from build123d import *

# Parameters (mm, degrees)
ESQUISSE1_W             = 23
ESQUISSE1_H             = 12
BOSS_EXTRU_1_DEPTH      = 21
ESQUISSE2_W             = 4
ESQUISSE2_H             = 11.992585314
BOSS_EXTRU_2_DEPTH      = 1
ESQUISSE3_R             = 0.5
ENL_V_MAT_EXTRU_1_DEPTH = 1
ESQUISSE4_R             = 5.976429807
BOSS_EXTRU_3_DEPTH      = 4
ESQUISSE5_W             = 4.5
ESQUISSE5_H             = 5
BOSS_EXTRU_4_DEPTH      = 3
ENL_V_MAT_EXTRU_3_DEPTH = 32.768695283
ESQUISSE7_R             = 1.5
ENL_V_MAT_EXTRU_4_DEPTH = 3


with BuildPart() as part:
    # Esquisse1 → Boss.-Extru.1 (new body)
    with BuildSketch(Plane(origin=(0, 0, 0), x_dir=(1, 0, 0), z_dir=(0, 1, 0))):
        Rectangle(ESQUISSE1_W, ESQUISSE1_H)
    extrude(amount=BOSS_EXTRU_1_DEPTH)

    # Esquisse2 → Boss.-Extru.2 (add)
    with BuildSketch(Plane(origin=(0, 16, 0), x_dir=(1, 0, 0), z_dir=(0, 1, 0))):
        with Locations((13.5, 0.003707343)):
            Rectangle(ESQUISSE2_W, ESQUISSE2_H)
    boss_extru_2 = extrude(amount=BOSS_EXTRU_2_DEPTH)

    # Esquisse3 → Enlèv. mat.-Extru.1 (cut)
    with BuildSketch(Plane(origin=(0, 17, 0), x_dir=(1, 0, 0), z_dir=(0, 1, 0))):
        with Locations(Location((13.5, 0.003707343, 0), (0, 0, 270))):
            Circle(ESQUISSE3_R)
    enl_v_mat_extru_1 = extrude(amount=-ENL_V_MAT_EXTRU_1_DEPTH, mode=Mode.SUBTRACT)

    # Symétrie1: Boss.-Extru.2 across plane
    add(boss_extru_2.mirror(Plane(origin=(0, 0, 0), x_dir=(0, 0, 1), z_dir=(1, 0, 0))))

    # Symétrie2: Enlèv. mat.-Extru.1 across plane
    add(enl_v_mat_extru_1.mirror(Plane(origin=(0, 0, 0), x_dir=(0, 0, 1), z_dir=(1, 0, 0))), mode=Mode.SUBTRACT)

    # Esquisse4 → Boss.-Extru.3 (add)
    with BuildSketch(Plane(origin=(0, 21, 0), x_dir=(1, 0, 0), z_dir=(0, 1, 0))):
        with Locations(Location((5.523570193, -0.023570193, 0), (0, 0, 270))):
            Circle(ESQUISSE4_R)
    extrude(amount=BOSS_EXTRU_3_DEPTH)

    # Esquisse5 → Boss.-Extru.4 (add)
    with BuildSketch(Plane(origin=(0, 21, 0), x_dir=(1, 0, 0), z_dir=(0, 1, 0))):
        with Locations((-0.452859613, -0.023570193)):
            Rectangle(ESQUISSE5_W, ESQUISSE5_H)
    extrude(amount=BOSS_EXTRU_4_DEPTH)

    # Esquisse6 → Enlèv. mat.-Extru.3 (cut, through all)
    with BuildSketch(Plane.XY.offset(6)):
        Polygon((9.55941942, 0), (11.5, 1.94058058), (11.5, 0), align=None)
    extrude(amount=-ENL_V_MAT_EXTRU_3_DEPTH, mode=Mode.SUBTRACT)

    # Esquisse7 → Enlèv. mat.-Extru.4 (cut)
    with BuildSketch(Plane(origin=(0, 25, 0), x_dir=(1, 0, 0), z_dir=(0, 1, 0))):
        with Locations(Location((5.523570193, -0.023570193, 0), (0, 0, 270))):
            Circle(ESQUISSE7_R)
    extrude(amount=-ENL_V_MAT_EXTRU_4_DEPTH, mode=Mode.SUBTRACT)


solid = part.part
Source: CAD feature listing. Evaluate the final solid. Frame: model axes, mm. A direction names the side the tool comes from. Give positions to 0.01 mm unless a question says otherwise; leave off trailing zeros. Write each loop counter-clockwise with the first axis right and the second up, starting at its lowest first coordinate (ties: lowest second). Pieces come first, ordered by that corner, then holes. Notation, with made-up numbers: M 24.5,-9.5 L 32.5,-9.5 A20 ccw 32.5,-2.5 Z; hole C -13,-1.5 d2. An arc over 180 degrees is marked long. Return JSON: item names as keys, results as strings. Group by question number.
1) Cut plane B-B, the plane z = -3.75. Output: boundary loops of the cut face in (x, y).
2) Ray query, L1, parallel to Z at x = -13.5, y = 16.5; L2, parallel to Y at x = 5.5, z = -1; L3, parallel to Y at x = -8, z = 1.5. Return the intervals inside material, ascending.
3) Cut plane D-D, the plane y = 10.25. Output: boundary loops of the cut face in (x, z), then the cut area to 3 significant figures.
4) Cut plane C-C, the plane x = 12. Output: boundary loops of the cut face in (y, z), then the cut area to 3 significant figures.
5) First-contact query: pin 1 Ø1 at (x, z) = (-6, 2) entering from +Y; pin 2 Ø0.8 at (x, z) = (-1.5, 0) entering from +Y; pin 3 Ø0.9 at (x, z) = (5.5, 0.5) entering from +Y. Flat tips, straight axial feed; report the tip coordinate or a pass-through.
6) Cut plane A-A, the plane x = -13.5. Output: boundary loops of the cut face in (y, z), then the cut area to 3 significant figures.
7) Set-up query: faces 1 (the face through (-11.5, 10, 0)), 2 (the face through (10.56, 22.97, 3.24)), 3 (the face through (-1, 22, -2.476)), 4 (the face through (11.5, 11, 0)). Return all of +Z, -Z, +X, -X, +Y, -Y with unobstructed straight access to the full face (end or side cutting, diameter ignored); none if empty.
8) Draft query along X for faces 5 (the face through (-13.996, 16.507, -0.069)), 6 (the face through (-14.4, 17, -0.1)), 7 (the face through (-2.703, 22, 0)). Return one class per face: released by +X, released by -X, zero draft, split by the parting line, or undercut.
Data:
{
 "1": {"outline": "M -15.5,16 L -11.5,16 L -11.5,0 L 9.56,0 L 11.5,1.94 L 11.5,16 L 15.5,16 L 15.5,17 L 11.5,17 L 11.5,21 L 10.16,21 L 10.16,25 L 0.89,25 L 0.89,21 L -11.5,21 L -11.5,17 L -15.5,17 Z"},
 "2": {"L1": "z = -6 to -0.5, 0.5 to 5.99", "L2": "y = 0 to 22", "L3": "y = 0 to 21"},
 "3": {"outline": "M -11.5,-6 L 11.5,-6 L 11.5,6 L -11.5,6 Z", "area": "276 mm²"},
 "4": {"outline": "M 16,-6 L 17,-6 L 17,5.99 L 16,5.99 Z", "area": "12.0 mm²"},
 "5": {"pin 1": "stops at y = 21", "pin 2": "stops at y = 24", "pin 3": "stops at y = 22"},
 "6": {"outline": "M 16,-6 L 17,-6 L 17,-0.5 L 16,-0.5 Z; M 16,0.5 L 17,0.5 L 17,5.99 L 16,5.99 Z", "area": "11.0 mm²"},
 "7": {"face 1": "+Z, -Z, -X", "face 2": "+Y", "face 3": "-Z, -X, +Y", "face 4": "+Z, -Z, +X"},
 "8": {"face 5": "undercut", "face 6": "zero draft", "face 7": "released by -X"}
}
